Geometry check sheet. Reference: the model listing, model coordinates, mm. Round coordinates to 2 decimals unless told otherwise and drop trailing zeros. Order: outer loops, then holes, each group sorted by start corner. A loop starts at its lowest first (then second) coordinate and runs counter-clockwise, first axis right, second up. Notation, with made-up numbers: (84.5, -33) -> (105.5, -33) arc R21 cw to (105.5, -21) -> close; hole circle Ø6 at (76, 47). An arc over 180 degrees is marked (long way). Answer as a JSON object with one key per item and string values. Group by question number.
from build123d import *

# Parameters (mm, degrees)
SKETCH1_R             = 82.5
BOSS_EXTRUDE1_DEPTH   = 3
F_3_0MM_DOWEL_HOLE1_D = 3
CIRPATTERN1_COUNT     = 5
SKETCH4_R             = 8
CUT_EXTRUDE1_DEPTH    = 117.711181984


with BuildPart() as part:
    # Sketch1 → Boss-Extrude1 (new body)
    with BuildSketch(Plane.XY):
        Circle(SKETCH1_R)
    extrude(amount=BOSS_EXTRUDE1_DEPTH)

    # Ø3.0mm Dowel Hole1 (through all)
    with Locations(Plane(origin=(0, 80, 3), x_dir=(1, 0, 0), z_dir=(0, 0, 1))):
        with Locations((0, 0)):
            f_3_0mm_dowel_hole1 = Hole(F_3_0MM_DOWEL_HOLE1_D / 2)

    # CirPattern1: Ø3.0mm Dowel Hole1 ×5 about axis
    cirpattern1_axis = Axis((0, 0, 0), (0, 0, 1))
    for i in range(1, CIRPATTERN1_COUNT):
        add(f_3_0mm_dowel_hole1.rotate(cirpattern1_axis, i * 360 / CIRPATTERN1_COUNT), mode=Mode.SUBTRACT)

    # Sketch4 → Cut-Extrude1 (cut, through all)
    with BuildSketch(Plane.XY.offset(3)):
        with Locations((15, 0)):
            Circle(SKETCH4_R)
    extrude(amount=-CUT_EXTRUDE1_DEPTH, mode=Mode.SUBTRACT)


solid = part.part
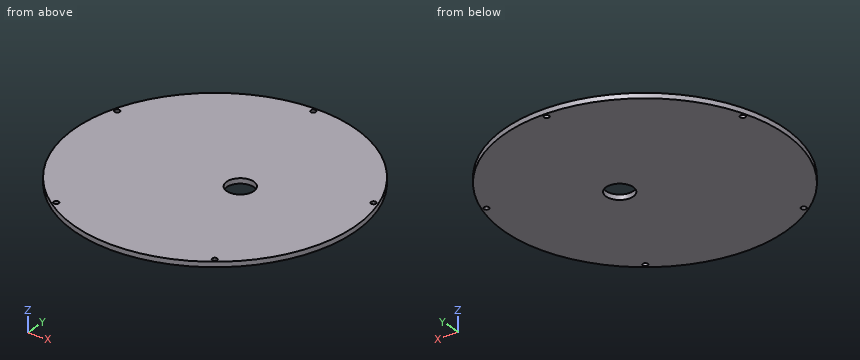
Item 1: Depth check by flat-ended pin: pin 1 Ø1.5 at (y, z) = (-52.5, 2.5) entering from -X. Enter the tip coordinate at first touch or a pass-through.
Item 2: Thickness scan on L1, parallel to Y at x = 15, z = 1.55; L2, parallel to Y at x = 2, z = 1.6; L3, parallel to Y at x = 21, z = 2. Record the ranges inside material, lowest first.
Item 3: Sectioned sample at A-A, the plane x = 15. Enter the section's corners in (y, z).
Item 4: Sectioned sample at C-C, the plane y = 60. Enter the section's corners in (x, z).
Item 5: Sectioned sample at D-D, the plane x = 61.5. Enter the section's corners in (y, z).
Item 6: Sectioned sample at B-B, the plane z = 1.1. Enter the section's corners in (x, y), then the cut area to 3 significant figures.
Result:
{
 "1": {"pin 1": "stops at x = -64.25"},
 "2": {"L1": "y = -81.12 to -8, 8 to 81.12", "L2": "y = -82.48 to 82.48", "L3": "y = -79.78 to -5.29, 5.29 to 79.78"},
 "3": {"outline": "(-81.12, 0) -> (-8, 0) -> (-8, 3) -> (-81.12, 3) -> close; (8, 0) -> (81.12, 0) -> (81.12, 3) -> (8, 3) -> close"},
 "4": {"outline": "(-56.62, 0) -> (56.62, 0) -> (56.62, 3) -> (-56.62, 3) -> close"},
 "5": {"outline": "(-54.99, 0) -> (54.99, 0) -> (54.99, 3) -> (-54.99, 3) -> close"},
 "6": {"outline": "circle Ø165 at (0, 0); hole circle Ø3 at (-76.08, 24.72); hole circle Ø3 at (-47.02, -64.72); hole circle Ø3 at (0, 80); hole circle Ø16 at (15, 0); hole circle Ø3 at (47.02, -64.72); hole circle Ø3 at (76.08, 24.72)", "area": "21,100 mm2"}
}
